Geometry: see drawing. Coordinates: mm, zero at the bounding-box minimum. A direction names the side the tool comes from. Coordinates: 2 decimals unless noted, no trailing zeros. Write each loop counter-clockwise with the first axis right and the second up, starting at its lowest first coordinate (ties: lowest second). Pieces come first, ordered by that corner, then holes.
1) Section query B-B (z = 2.75). Output: boundary loops of the cut face in (x, y) (1 decimal).
2) Line query: L1, parallel to Y at x = 21, z = 5.25 (1 decimal); L2, parallel to X at y = 30.5, z = 7; L3, parallel to X at y = 88.5, z = 9.5 (1 decimal). Output: solid intervals per line, ascending.
3) Section query A-A (y = 5). Output: boundary loops of the cut face in (x, z).
4) Section query C-C (y = 70). Output: boundary loops of the cut face in (x, z).
5) Set-up query: the marked faces 1, 2 and 3. Return all of +Z, -Z, +X, -X, +Y, -Y with unobstructed straight access to the full face (end or side cutting, diameter ignored); none if empty.
6) Section query D-D (y = 15.5). Output: boundary loops of the cut face in (x, z), then the cut area to 3 significant figures.
7) Pin query (flat end, axial travel): pin 1 Ø6 at (x, z) = (16.5, 1.5) entering from +Y (1 decimal); pin 2 Ø1.9 at (x, z) = (4.5, 4.5) entering from +Y (1 decimal); pin 3 Ø3.5 at (x, y) = (4.33, 19.33) entering from -Z; pin 4 Ø5 at (y, z) = (29.5, 2.5) entering from -X. Return the tip coordinate at first contact, or that it passes through.
8) Draft query along Y for the marked faces 4, 5 and 6. Return one class per face: pulls with the +Y half, pulls with the -Y half, needs draft (parallel to the pull), parting line crosses it, or undercut.
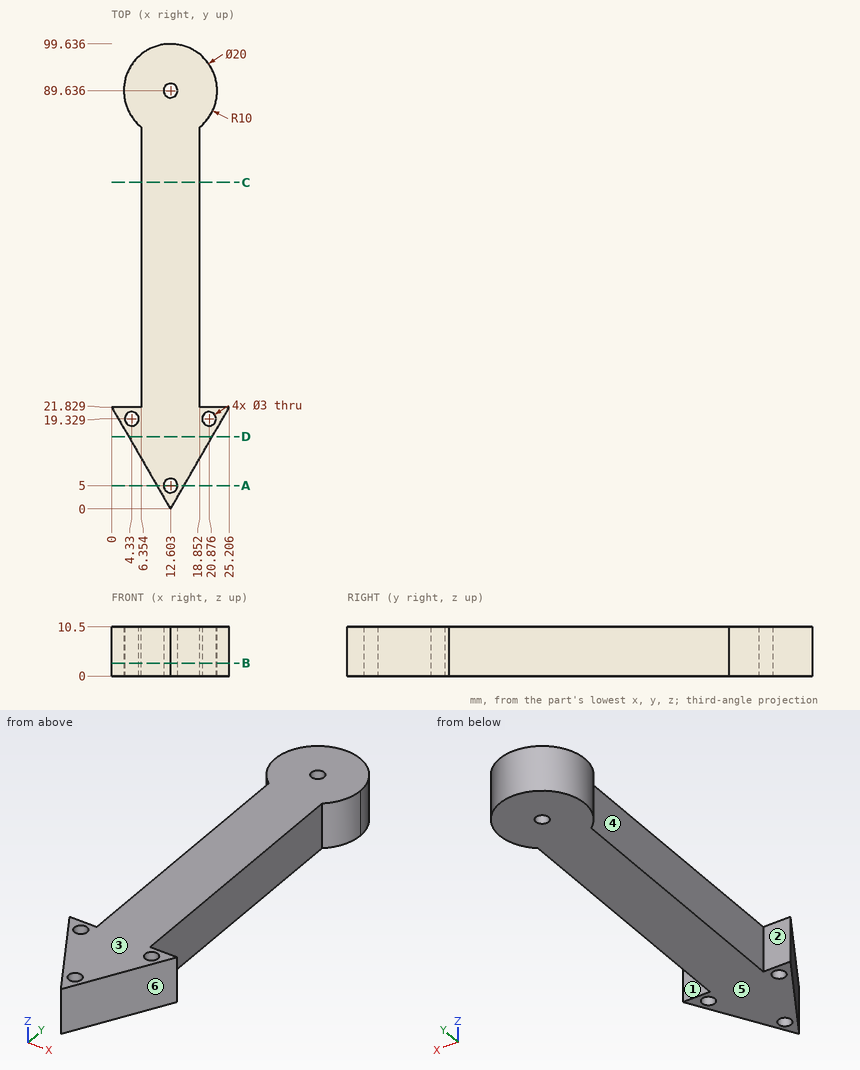
Answer:
1. outline: (0, 21.8) - (12.6, 0) - (25.2, 21.8) - (18.9, 21.8) - (18.9, 81.8) arc R10 ccw to (22.6, 89.6) arc R10 ccw (long way) to (6.4, 81.8) - (6.4, 21.8) - close; hole circle Ø3 at (4.3, 19.3); hole circle Ø3 at (12.6, 5); hole circle Ø3 at (12.6, 89.6); hole circle Ø3 at (20.9, 19.3)
2. L1: y = 14.5 to 17.8, 20.8 to 21.8, 84.2 to 95.1
2. L2: x = 6.35 to 18.85
2. L3: x = 2.7 to 11.6, 13.6 to 22.5
3. outline: (9.72, 0) - (11.1, 0) - (11.1, 10.5) - (9.72, 10.5) - close; (14.1, 0) - (15.49, 0) - (15.49, 10.5) - (14.1, 10.5) - close
4. outline: (6.35, 0) - (18.85, 0) - (18.85, 10.5) - (6.35, 10.5) - close
5. face 1: +Z, -Z, +X
5. face 2: +Z, -Z, -X
5. face 3: +Z, +X, -X, +Y, -Y
6. outline: (3.65, 0) - (21.55, 0) - (21.55, 10.5) - (3.65, 10.5) - close
6. area: 188 mm2
7. pin 1: stops at y = 99.6
7. pin 2: stops at y = 96.6
7. pin 3: stops at z = 0
7. pin 4: stops at x = 6.35
8. face 4: undercut
8. face 5: needs draft
8. face 6: pulls with the -Y half
